Verification items for the finished model (mm, model axes). Face numbers are marked on the shaded views. A direction names the side the tool comes from. Coordinates: 2 decimals unless noted, no trailing zeros. Loops run counter-clockwise (first coordinate to the right, second up) from the corner with the lowest first, then second, coordinate; pieces in that order, holes last. Notation, with made-up numbers: M 40.5,11.5 L 94.5,11.5 A36 cw 94.5,47.5 Z; hole C 6.5,-22 d5. An arc over 180 degrees is marked long. Write item = value, one per line. Start each with the question number.
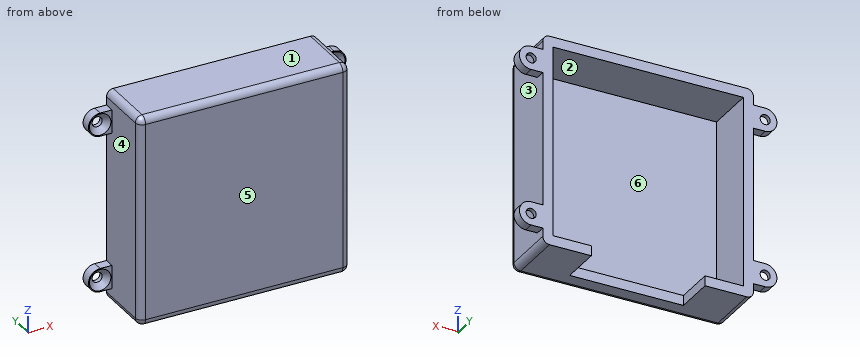
```python
from build123d import *

# Parameters (mm, degrees)
SKETCH1_W           = 63
SKETCH1_H           = 63
BOSS_EXTRUDE1_DEPTH = 18
SHELL2_T            = -3
SKETCH2_W           = 34
SKETCH2_H           = 12
CUT_EXTRUDE1_DEPTH  = 3
FILLET2_R           = 2
SKETCH4_R           = 1.5
BOSS_EXTRUDE2_DEPTH = 3
CHAMFER1_SIZE       = 1.7


with BuildPart() as part:
    # Sketch1 → Boss-Extrude1 (new body)
    with BuildSketch(Plane(origin=(0, 0, 0), x_dir=(1, 0, 0), z_dir=(0, 1, 0))):
        with Locations((31.5, 31.5)):
            Rectangle(SKETCH1_W, SKETCH1_H)
    extrude(amount=BOSS_EXTRUDE1_DEPTH)

    # Shell2
    shell2_openings = [part.faces().sort_by_distance(p)[0] for p in [
        (31.5, 18, -31.5),
    ]]
    offset(amount=SHELL2_T, openings=shell2_openings, kind=Kind.INTERSECTION)

    # Sketch2 → Cut-Extrude1 (cut)
    with BuildSketch(Plane(origin=(0, 0, -63), x_dir=(-1, 0, 0), z_dir=(0, 0, -1))):
        with Locations((-31.5, 12)):
            Rectangle(SKETCH2_W, SKETCH2_H)
    extrude(amount=-CUT_EXTRUDE1_DEPTH, mode=Mode.SUBTRACT)

    # Fillet2
    fillet2_edges = [part.edges().sort_by_distance(p)[0] for p in [
        (31.5, 0, -63),
        (63, 0, -31.5),
        (31.5, 0, 0),
        (0, 0, -31.5),
        (0, 9, -63),
        (63, 9, -63),
        (63, 9, 0),
        (0, 9, 0),
    ]]
    fillet(fillet2_edges, radius=FILLET2_R)

    # Sketch4 → Boss-Extrude2 (add)
    # profile 1 of 4: a face of its own
    with BuildSketch(Plane(origin=(0, 18, 0), x_dir=(1, 0, 0), z_dir=(0, 1, 0))):
        with BuildLine():
            Line((0, 58.5), (0, 51.5))
            Line((0, 51.5), (-3.5, 51.5))
            ThreePointArc((-3.5, 51.5), (-7, 55), (-3.5, 58.5))
            Line((-3.5, 58.5), (0, 58.5))
        make_face()
        with Locations(Location((-3.5, 55, 0), (0, 0, 270))):
            Circle(SKETCH4_R, mode=Mode.SUBTRACT)
    # profile 2 of 4: a face of its own
    with BuildSketch(Plane(origin=(0, 18, 0), x_dir=(1, 0, 0), z_dir=(0, 1, 0))):
        with BuildLine():
            Line((66.5, 51.5), (63, 51.5))
            Line((63, 51.5), (63, 58.5))
            Line((63, 58.5), (66.5, 58.5))
            ThreePointArc((66.5, 58.5), (70, 55), (66.5, 51.5))
        make_face()
        with Locations(Location((66.5, 55, 0), (0, 0, 90))):
            Circle(SKETCH4_R, mode=Mode.SUBTRACT)
    # profile 3 of 4: a face of its own
    with BuildSketch(Plane(origin=(0, 18, 0), x_dir=(1, 0, 0), z_dir=(0, 1, 0))):
        with BuildLine():
            Line((63, 4.5), (63, 11.5))
            Line((63, 11.5), (66.5, 11.5))
            ThreePointArc((66.5, 11.5), (70, 8), (66.5, 4.5))
            Line((66.5, 4.5), (63, 4.5))
        make_face()
        with Locations(Location((66.5, 8, 0), (0, 0, 270))):
            Circle(SKETCH4_R, mode=Mode.SUBTRACT)
    # profile 4 of 4: a face of its own
    with BuildSketch(Plane(origin=(0, 18, 0), x_dir=(1, 0, 0), z_dir=(0, 1, 0))):
        with BuildLine():
            Line((-3.5, 11.5), (0, 11.5))
            Line((0, 11.5), (0, 4.5))
            Line((0, 4.5), (-3.5, 4.5))
            ThreePointArc((-3.5, 4.5), (-7, 8), (-3.5, 11.5))
        make_face()
        with Locations(Location((-3.5, 8, 0), (0, 0, 90))):
            Circle(SKETCH4_R, mode=Mode.SUBTRACT)
    extrude(amount=-BOSS_EXTRUDE2_DEPTH)

    # Chamfer1
    chamfer1_edges = [part.edges().sort_by_distance(p)[0] for p in [
        (66.5, 15, -9.5),
        (-3.5, 15, -6.5),
        (-3.5, 15, -56.5),
        (66.5, 15, -53.5),
    ]]
    chamfer(chamfer1_edges, length=CHAMFER1_SIZE)


solid = part.part
```
Q1. Set-up check for the marked faces 1 and 2: record each of +Z, -Z, +X, -X, +Y, -Y from which the full face is reachable in a straight line by a thin tool's end or side.
Q2. Sectioned sample at C-C on x = 58.5. Record the cut outline in (y, z).
Q3. Gauge pin test, flat ends, axial feed: pin 1 (8 mm diameter, centred on x = 26.5, y = 15, fed in from -Z); pin 2 (7.5 mm diameter, centred on x = -3, z = -55, fed in from -Y); pin 3 (3 mm diameter, centred on y = 4, z = -21.5, fed in from +X). Record the tip position at first contact, or that the pin passes through.
Q4. Sectioned sample at A-A on z = -55. Record the cut outline in (x, y), plus the area to 3 significant figures.
Q5. Sectioned sample at B-B on y = 7.75. Record the cut outline in (x, z), plus the area to 3 significant figures.
Q6. Scan lines: L1, parallel to Z at x = 66.5, y = 17.55; L2, parallel to X at y = 17.1, z = -55; L3, parallel to Z at x = 12, y = 11.25. Record each from-to range of solid material in increasing order. Write a range as [from, to].
Q7. Mould release check, pull along X, two halves, no side actions. Record for the marked faces 3, 4, 5 and 6: +X half, -X half, draft (parallel to the pull), parting line (faces both ways), or undercut.
Q8. Sectioned sample at D-D on z = -15. Record the cut outline in (x, y).
Solutions:
q1.face_1 = +Z, +X, -X, +Y, -Y
q1.face_2 = +Y
q2.outline = M 0,-61 A2 ccw 2,-63 L 18,-63 L 18,-60 L 3,-60 L 3,-3 L 18,-3 L 18,0 L 2,0 A2 ccw 0,-2 Z
q3.pin_1 = -3
q3.pin_2 = 0.44
q3.pin_3 = 63
q4.outline = M -7,15 L -6.7,15 L -5,16.7 L -5,18 L -7,18 Z; M -2,16.7 L -0.3,15 L 0,15 L 0,2 A2 ccw 2,0 L 61,0 A2 ccw 63,2 L 63,15 L 63.3,15 L 65,16.7 L 65,18 L 60,18 L 60,3 L 3,3 L 3,18 L -2,18 Z; M 68,16.7 L 69.7,15 L 70,15 L 70,18 L 68,18 Z
q4.area = 296 mm²
q5.outline = M 0,-61 A2 ccw 2,-63 L 14.5,-63 L 14.5,-60 L 3,-60 L 3,-3 L 60,-3 L 60,-60 L 48.5,-60 L 48.5,-63 L 61,-63 A2 ccw 63,-61 L 63,-2 A2 ccw 61,0 L 2,0 A2 ccw 0,-2 Z
q5.area = 615 mm²
q6.L1 = [-58.5, -56.5], [-53.5, -51.5], [-11.5, -9.5], [-6.5, -4.5]
q6.L2 = [-7, -5], [-2, 3], [60, 65], [68, 70]
q6.L3 = [-63, -60], [-3, 0]
q7.face_3 = +X half
q7.face_4 = -X half
q7.face_5 = draft
q7.face_6 = undercut
q8.outline = M 0,2 A2 ccw 2,0 L 61,0 A2 ccw 63,2 L 63,18 L 60,18 L 60,3 L 3,3 L 3,18 L 0,18 Z
